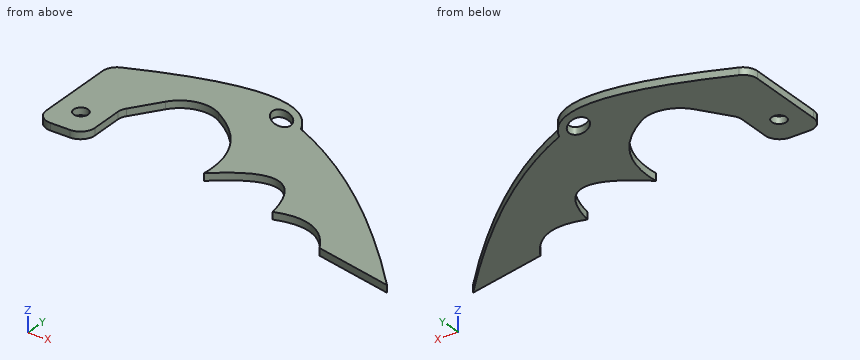
```python
from build123d import *

# Parameters (mm, degrees)
SKETCH1_R           = 3.175
SKETCH1_RX          = 6.501731069
SKETCH1_RY          = 3.917709747
BOSS_EXTRUDE1_DEPTH = 3.175
FILLET1_R           = 6.35
FILLET2_R           = 15.24
FILLET3_R           = 6.35


with BuildPart() as part:
    # Sketch1 → Boss-Extrude1 (new body)
    with BuildSketch(Plane.XY):
        with BuildLine():
            Line((85.837990546, -35.686780557), (50.815428811, -28.169433219))
            add(Edge.make_bspline(
                [(22.151507794, -16.88306006), (40.93348508, -10.477937426), (50.815428811, -28.169433219)],
                knots=[0, 0, 0, 1, 1, 1], degree=2))
            add(Edge.make_bspline(
                [(-13.89812039, -8.73455109), (16.354395889, 17.832088288), (22.151507794, -16.88306006)],
                knots=[0, 0, 0, 1, 1, 1], degree=2))
            add(Edge.make_bspline(
                [(-47.440785313, 35.367440163), (-10.94231892, 21.565916132), (-13.89812039, -8.73455109)],
                knots=[0, 0, 0, 1, 1, 1], degree=2))
            Line((-47.440785313, 35.367440163), (-64.461456133, 11.041010118))
            Line((-64.461456133, 11.041010118), (-64.461456133, -11.388692522))
            Line((-64.461456133, -11.388692522), (-85.837990546, -11.388692522))
            Line((-85.837990546, -11.388692522), (-85.837990546, 33.806971222))
            add(Edge.make_bspline(
                [(-85.837990546, 33.806971222), (-15.708828484, 64.705105309), (-3.996524698, 37.11343766)],
                knots=[0, 0, 0, 0.406769717, 0.406769717, 0.406769717], degree=2))
            add(Edge.make_bspline(
                [(85.837990546, -35.686780557), (37.045439563, 18.631346841), (-3.996524698, 37.11343766)],
                knots=[0, 0, 0, 0.371923551, 0.371923551, 0.371923551], degree=2))
        make_face()
        with Locations((-75.14972334, 1.323731685)):
            Circle(SKETCH1_R, mode=Mode.SUBTRACT)
        with Locations(Location((-14.065908589, 39.346528079), (0, 0, 142.125016349))):
            Ellipse(SKETCH1_RX, SKETCH1_RY, mode=Mode.SUBTRACT)
    extrude(amount=BOSS_EXTRUDE1_DEPTH)

    # Fillet1
    fillet1_edges = [part.edges().sort_by_distance(p)[0] for p in [
        (-64.461456133, 11.041010118, 1.5875),
        (-64.461456133, -11.388692522, 1.5875),
        (-85.837990546, -11.388692522, 1.5875),
    ]]
    fillet(fillet1_edges, radius=FILLET1_R)

    # Fillet2
    fillet2_edges = [part.edges().sort_by_distance(p)[0] for p in [
        (-47.440785313, 35.367440163, 1.5875),
    ]]
    fillet(fillet2_edges, radius=FILLET2_R)

    # Fillet3
    fillet3_edges = [part.edges().sort_by_distance(p)[0] for p in [
        (-85.837990546, 33.806971222, 1.5875),
    ]]
    fillet(fillet3_edges, radius=FILLET3_R)


solid = part.part
```
Here's how the part is built. I have some questions about the finished solid (model axes, mm). Coordinates: 2 decimals unless noted, no trailing zeros. Answer as a JSON object with one key per item and string values. Group by question number.
(1) I need wall thicknesses on probe 1 along X at (y, z) = (-2.5, 0.7); probe 2 along X at (y, z) = (20, 0.8); probe 3 along X at (y, z) = (36, 2.8). Which ranges of each line are inside material? Lowest first, please.
(2) Suppose I cut it at A-A, the plane y = -7. State how many separate pieces and enclosed holes the cut face has, then the cut area to 3 significant figures.
(3) For pin 1 (1.5 mm diameter, centred on y = -24.5, z = 3, fed in from -X); pin 2 (1 mm diameter, centred on x = 40.5, z = 2.5, fed in from -Y); pin 3 (1 mm diameter, centred on y = 4, z = 2.5, fed in from +X), each with a flat end and sliding along its axis, tell me the tip position at first contact or that it passes through.
Values found:
{
 "1": {"probe 1": "x = -85.84 to -64.46, -13.71 to -5.91, 17.17 to 53.12", "probe 2": "x = -85.84 to -58.19, -22.94 to 25.38", "probe 3": "x = -80.76 to -16.13, -8.58 to -1.59"},
 "2": {"separate pieces": "3", "enclosed holes": "0", "area": "194 mm^2"},
 "3": {"pin 1": "stops at x = 47.92", "pin 2": "stops at y = -17.59", "pin 3": "stops at x = 46.36"}
}
